For this review, take the finished solid that the model builds, in its own axes (mm). A direction names the side the tool comes from. Coordinates: 2 decimals unless noted, no trailing zeros. Loops run counter-clockwise (first coordinate to the right, second up) from the corner with the lowest first, then second, coordinate; pieces in that order, holes last.
1. Clearance check with flat-ended pins moving along their axes: P1, Ø3.5, axis at y = 72.5, z = -57.5, coming from the +X side; P2, Ø5, axis at x = -10, y = 73.5, coming from the +Z side; P3, Ø8, axis at x = -3.5, y = 73, coming from the -Z side. State where each tip first meets the part, or that it passes through.
2. Take a section at A-A, the plane x = 0. State the section outline as (y, z) points, then the cut area to 3 significant figures.
3. Take a section at D-D, the plane y = -14.5. State the section outline as (x, z) points.
4. Take a section at B-B, the plane z = -11. State the section outline as (x, y) points, then the cut area to 3 significant figures.
5. Take a section at C-C, the plane z = 69. State the section outline as (x, y) points, then the cut area to 3 significant figures.
6. Machinability: for faces 4 (the face through (-80, -12, 15)), 5 (the face through (-83, -12, 15)), 6 (the face through (-8, 73, 35)), 7 (the face through (-22, 71.887, 1)), 8 (the face through (-8, 73, -35)), which of the approach directions +Z, -Z, +X, -X, +Y, -Y give a long, thin tool a straight path to every point of the face, cutting with its end or side? Answer none if there is none.
7. Mouldability with a two-part tool opening along Y and no side actions: class faces 1 (the face through (3.997, 73.232, 0.49)), 2 (the face through (-70.738, 61.956, 14.717)), 3 (the face through (-95, -68.113, 27)) as pulls with the +Y half, pulls with the -Y half, needs draft (parallel to the pull), parting line crosses it, or undercut.
8. To check wall thickness, follow probe 1 along Y at (x, z) = (0, -9.5); probe 2 along Y at (x, z) = (-19.5, -15); probe 3 along X at (y, z) = (-22, -8). State the ranges of each line that lie inside material, in increasing order.
```python
from build123d import *

# Parameters (mm, degrees)
BOSS_EXTRUDE2_DEPTH = 105
SKETCH2_W           = 40
SKETCH2_H           = 70
CUT_EXTRUDE1_DEPTH  = 105
FILLET1_R           = 20
FILLET2_R           = 20
SKETCH3_R           = 5
SKETCH3_R_2         = 4
BOSS_EXTRUDE3_DEPTH = 70
SKETCH4_R           = 3.960689981
CUT_EXTRUDE2_DEPTH  = 70
SKETCH5_W           = 109.66717185
SKETCH5_H           = 31.212047829
CUT_EXTRUDE3_DEPTH  = 226.995575224
FILLET3_R           = 20
CUT_EXTRUDE4_DEPTH  = 228.140735518


with BuildPart() as part:
    # Sketch1 → Boss-Extrude2 (new, symmetric)
    with BuildSketch(Plane.XY):
        with BuildLine():
            Line((0, 71.886792453), (-40, 71.886792453))
            ThreePointArc((-40, 71.886792453), (-68.284271247, 60.1710637), (-80, 31.886792453))
            Line((-80, 31.886792453), (-80, -58.113207547))
            ThreePointArc((-80, -58.113207547), (-82.928932188, -65.184275359), (-90, -68.113207547))
            Line((-90, -68.113207547), (-140, -68.113207547))
            Line((-140, -68.113207547), (-94.515046268, -67.122597845))
            ThreePointArc((-94.515046268, -67.122597845), (-93.499760174, -67.04866017), (-92.497251559, -66.871885994))
            Line((-92.497251559, -66.871885994), (-91.47680263, -66.637838075))
            ThreePointArc((-91.47680263, -66.637838075), (-87.662546027, -64.853336369), (-84.921098336, -61.656859506))
            Line((-84.921098336, -61.656859506), (-84.208764192, -60.34289018))
            ThreePointArc((-84.208764192, -60.34289018), (-83.306900442, -58.035369732), (-83, -55.576951347))
            Line((-83, -55.576951347), (-83, 31.886792453))
            ThreePointArc((-83, 31.886792453), (-70.405591591, 62.292384044), (-40, 74.886792453))
            Line((-40, 74.886792453), (0, 74.886792453))
            Line((0, 74.886792453), (0, 71.886792453))
        make_face()
    extrude(amount=BOSS_EXTRUDE2_DEPTH, both=True)

    # Sketch2 → Cut-Extrude1 (cut, symmetric)
    with BuildSketch(Plane(origin=(0, 74.886792453, 0), x_dir=(1, 0, 0), z_dir=(0, 1, 0))):
        with Locations((-20, 70)):
            Rectangle(SKETCH2_W, SKETCH2_H)
        with Locations((-20, -70)):
            Rectangle(SKETCH2_W, SKETCH2_H)
    extrude(amount=CUT_EXTRUDE1_DEPTH, both=True, mode=Mode.SUBTRACT)

    # Fillet1
    fillet1_edges = [part.edges().sort_by_distance(p)[0] for p in [
        (-40, 73.386792453, -35),
        (-40, 73.386792453, 35),
    ]]
    fillet(fillet1_edges, radius=FILLET1_R)

    # Fillet2
    # the kernel refuses this fillet: 20 mm, written as the material it takes off along each edge
    with BuildSketch(Plane(origin=(-40, 21.886792453, -105), x_dir=(-1, 0, 0), z_dir=(0, 1, 0)), Plane(origin=(-40, 124.886792453, 105), x_dir=(-1, 0, 0), z_dir=(0, -1, 0))) as fillet2_piece_1:
        with BuildLine():
            CenterArc((FILLET2_R, FILLET2_R), FILLET2_R, 180, 90)
            Line((0, FILLET2_R), (0, 0))
            Line((0, 0), (FILLET2_R, 0))
        make_face()
    extrude(amount=103, mode=Mode.SUBTRACT)

    # Sketch3 → Boss-Extrude3 (add)
    with BuildSketch(Plane.XY.offset(35)):
        with Locations((0, 73.386792453)):
            Circle(SKETCH3_R)
        with Locations((0, 73.386792453)):
            Circle(SKETCH3_R_2, mode=Mode.SUBTRACT)
    extrude(amount=-BOSS_EXTRUDE3_DEPTH)

    # Sketch4 → Cut-Extrude2 (cut)
    with BuildSketch(Plane.XY.offset(35)):
        with Locations((0, 73.386792453)):
            Circle(SKETCH4_R)
    extrude(amount=-CUT_EXTRUDE2_DEPTH, mode=Mode.SUBTRACT)

    # Sketch5 → Cut-Extrude3 (cut, through all)
    with BuildSketch(Plane(origin=(0, 74.886792453, 0), x_dir=(1, 0, 0), z_dir=(0, 1, 0))):
        with Locations((-94.833585925, 93.735031647)):
            Rectangle(SKETCH5_W, SKETCH5_H)
    extrude(amount=-CUT_EXTRUDE3_DEPTH, mode=Mode.SUBTRACT)

    # Fillet3
    # the kernel refuses this fillet: 20 mm, written as the material it takes off along each edge
    with BuildSketch(Plane(origin=(-40, 124.886792453, -78.129007732), x_dir=(-1, 0, 0), z_dir=(0, -1, 0))) as fillet3_piece_1:
        with BuildLine():
            CenterArc((FILLET3_R, -FILLET3_R), FILLET3_R, 90, 90)
            Line((0, -FILLET3_R), (0, 0))
            Line((0, 0), (FILLET3_R, 0))
        make_face()
    extrude(amount=103, mode=Mode.SUBTRACT)

    # Sketch6 → Cut-Extrude4 (cut, through all)
    with BuildSketch(Plane(origin=(1.416350581, -65.033322939, 0), x_dir=(0.9997629253149604, 0.021773680572498965, 0), z_dir=(-0.021773680572498965, 0.9997629253149604, 0))):
        with BuildLine():
            Line((-141.449884768, 78.129007732), (-141.449884768, -105))
            ThreePointArc((-141.449884768, -105), (-96.291711515, -13.435496134), (-141.449884768, 78.129007732))
        make_face()
    extrude(amount=-CUT_EXTRUDE4_DEPTH, mode=Mode.SUBTRACT)


solid = part.part
```
Results list:
1. P1: stops at x = -40
1. P2: stops at z = 35
1. P3: stops at z = -35
2. outline: (68.39, -35) - (69.39, -35) - (69.39, 35) - (68.39, 35) - close; (77.39, -35) - (78.39, -35) - (78.39, 35) - (77.39, 35) - close
2. area: 140 mm2
3. outline: (-83, -78.13) - (-80, -78.13) - (-80, 105) - (-83, 105) - close
4. outline: (-97.47, -67.19) - (-97.45, -68.11) - (-90, -68.11) arc R10 ccw to (-80, -58.11) - (-80, 31.89) arc R40 cw to (-40, 71.89) - (-4.77, 71.89) arc R5 ccw (long way) to (-4.77, 74.89) - (-40, 74.89) arc R43 ccw to (-83, 31.89) - (-83, -55.58) arc R10 cw to (-84.21, -60.34) - (-84.92, -61.66) arc R10 cw to (-91.48, -66.64) - (-92.5, -66.87) arc R10 cw to (-94.52, -67.12) - close; hole (-3.71, 71.89) arc R4 ccw (long way) to (-3.71, 74.89) - (-3.67, 74.89) arc R3.96 ccw to (-3.67, 71.89) - close
4. area: 652 mm2
5. outline: (-109.11, -67.44) - (-109.09, -68.11) - (-90, -68.11) arc R10 ccw to (-80, -58.11) - (-80, 31.89) arc R40 cw to (-40, 71.89) - (-40, 74.89) arc R43 ccw to (-83, 31.89) - (-83, -55.58) arc R10 cw to (-84.21, -60.34) - (-84.92, -61.66) arc R10 cw to (-91.48, -66.64) - (-92.5, -66.87) arc R10 cw to (-94.52, -67.12) - close
5. area: 527 mm2
6. face 4: +Z, -Z, +X, -Y
6. face 5: +Z, -Z, -X, +Y
6. face 6: +Z, +X, +Y, -Y
6. face 7: +Z, -Z, -Y
6. face 8: -Z, +X, +Y, -Y
7. face 1: undercut
7. face 2: pulls with the +Y half
7. face 3: pulls with the -Y half
8. probe 1: y = 68.39 to 69.39, 77.39 to 78.39
8. probe 2: y = 71.89 to 74.89
8. probe 3: x = -83 to -80
